Job drawing, mm, ordinate dimensions from the low corner. One solid piece. Give positions to 0.01 mm unless a question says otherwise; leave off trailing zeros. Write each loop counter-clockwise with the first axis right and the second up, starting at its lowest first coordinate (ties: lowest second). Pieces come first, ordered by that corner, then holes. Notation, with made-up numbers: M 53,-27 L 86,-27 A6 cw 86,-20 Z; hole C 41.25,23.5 d10. An arc over 180 degrees is marked long. Answer as CSV lines item,"result". Start each with the question number.
Item 1: Band-saw the part on C-C, the plane y = 7. List the corners of the cut face in (x, z), then the cut area to 3 significant figures.
Item 2: Band-saw the part on B-B, the plane x = 5.75. List the corners of the cut face in (y, z) (1 decimal).
Item 3: Band-saw the part on A-A, the plane x = 2. List the corners of the cut face in (y, z) (1 decimal).
Item 4: Pin check, flat tip, straight feed: pin 1 (1 mm diameter, centred on y = 38.5, z = 1, fed in from -X). Stop position of the tip, or through.
Item 5: Wall check: L1, parallel to Z at x = 4, y = 6.5; L2, parallel to Y at x = 9, z = 0.45; L3, parallel to X at y = 39, z = 1.45. Give the ranges that are in metal, low to high. Write a range as from..to.
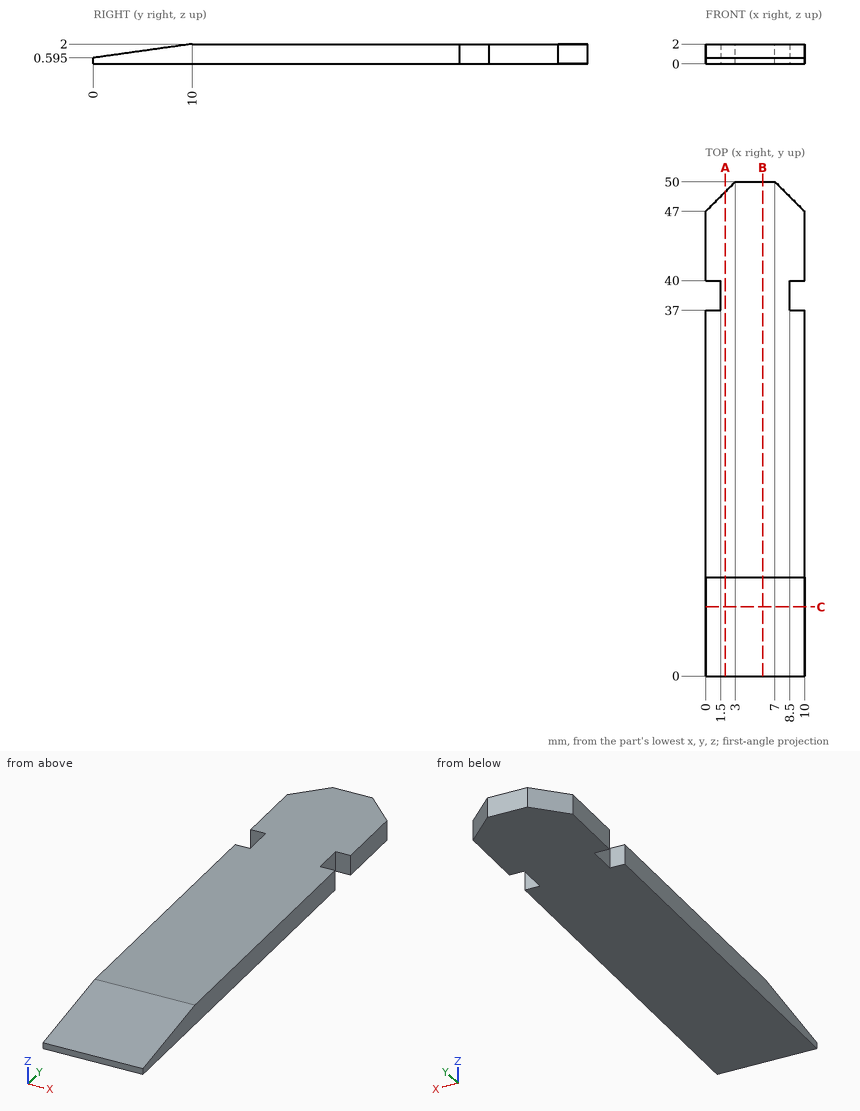
Output:
1,outline,"M 0,0 L 10,0 L 10,1.58 L 0,1.58 Z"
1,area,"15.8 mm²"
2,outline,"M 0,0 L 50,0 L 50,2 L 10,2 L 0,0.6 Z"
3,outline,"M 0,0 L 49,0 L 49,2 L 10,2 L 0,0.6 Z"
4,pin 1,"x = 1.5"
5,L1,"0..1.51"
5,L2,"0..37, 40..48"
5,L3,"1.5..8.5"
